Autodesk Inventor part; units mm, degrees
ref_plane "YZ Plane" through (0, 0, 0) normal (1, 0, 0) x (0, 1, 0)
ref_plane "XZ Plane" through (0, 0, 0) normal (0, 1, 0) x (-1, 0, 0)
ref_plane "XY Plane" through (0, 0, 0) normal (0, 0, 1) x (1, 0, 0)
sketch "Sketch1" plane through (0, 0, 0) normal (0, 1, 0) x (-1, 0, 0)
  line L0 (-21, 21) -> (21, 21)
  line L1 (21, 21) -> (21, -21)
  line L2 (21, -21) -> (-21, -21)
  line L3 (-21, -21) -> (-21, 21)
  line L4 (-21, 21) -> (21, -21) construction
  line L5 (21, 21) -> (-21, -21) construction
  point P0 (0, 0)
  dimension "d0" = 42
  dimension "d1" = 42
extrude "Extrusion1" add sketch "Sketch1" along normal blind 3
sketch "Sketch2" plane through (0, 3, 0) normal (0, 1, 0) x (1, 0, 0)
  circle A0 centre (0, 0) radius 3
  circle A1 centre (-15.5, -15.5) radius 1.8
  circle A2 centre (-15.5, 15.5) radius 1.8
  circle A3 centre (15.5, 15.5) radius 1.8
  circle A4 centre (15.5, -15.5) radius 1.8
  dimension "d4" = 6
  dimension "d5" = 3.6
  dimension "d6" = 31
  dimension "d7" = 15.5
  dimension "d8" = 15.5
  dimension "d9" = 31
extrude "Extrusion2" cut sketch "Sketch2" against normal blind 10
sketch "Sketch3" plane through (0, 3, 0) normal (0, 1, 0) x (1, 0, 0)
  circle A0 centre (-15.5, -15.5) radius 1.8
  circle A1 centre (-15.5, -15.5) radius 3.5
  circle A2 centre (0, 0) radius 19.3
  line L0 (-13.0251, -17.9749) -> (-10.946, -15.8958)
  line L1 (-17.9749, -13.0251) -> (-15.8958, -10.946)
  circle A3 centre (15.5, -15.5) radius 1.8
  circle A4 centre (15.5, -15.5) radius 3.5
  circle A5 centre (15.5, 15.5) radius 1.8
  circle A6 centre (15.5, 15.5) radius 3.5
  circle A7 centre (-15.5, 15.5) radius 1.8
  circle A8 centre (-15.5, 15.5) radius 3.5
  line L2 (13.0251, -17.9749) -> (10.946, -15.8958)
  line L3 (17.9749, -13.0251) -> (15.8958, -10.946)
  line L4 (13.0251, 17.9749) -> (10.946, 15.8958)
  line L5 (17.9749, 13.0251) -> (15.8958, 10.946)
  line L6 (-15.8958, 10.946) -> (-17.9749, 13.0251)
  line L7 (-10.946, 15.8958) -> (-13.0251, 17.9749)
  circle A9 centre (15.5, 15.5) radius 1.8
  circle A10 centre (-15.5, 15.5) radius 1.8
  circle A11 centre (15.5, -15.5) radius 1.8
  circle A12 centre (-15.5, -15.5) radius 1.8
  circle A13 centre (0, 0) radius 3
  line L8 (-21, 21) -> (-21, -21)
  line L9 (-21, -21) -> (21, -21)
  line L10 (21, -21) -> (21, 21)
  line L11 (21, 21) -> (-21, 21)
  dimension "d13" = 38.6
  dimension "d12" = 7
extrude "Extrusion3" cut sketch "Sketch3" against normal blind 10 contours L11 L10 L9 L8
sketch "Sketch4" plane through (0, 3, 0) normal (0, 1, 0) x (1, 0, 0)
  circle A0 centre (0, 0) radius 3
  circle A1 centre (0, 0) radius 16.125
  circle A2 centre (0, 0) radius 13.125
  dimension "d16" = 32.25
  dimension "d17" = 3
extrude "Extrusion4" add sketch "Sketch4" along normal blind 3 contours A1
fillet "Fillet1" radius 4 8 edges at (-15.8958, 1.5, -10.946) (-15.8958, 1.5, 10.946) (-10.946, 1.5, 15.8958) (10.946, 1.5, 15.8958) (15.8958, 1.5, 10.946) (15.8958, 1.5, -10.946) (10.946, 1.5, -15.8958) (-10.946, 1.5, -15.8958)
properties part number "Lid"
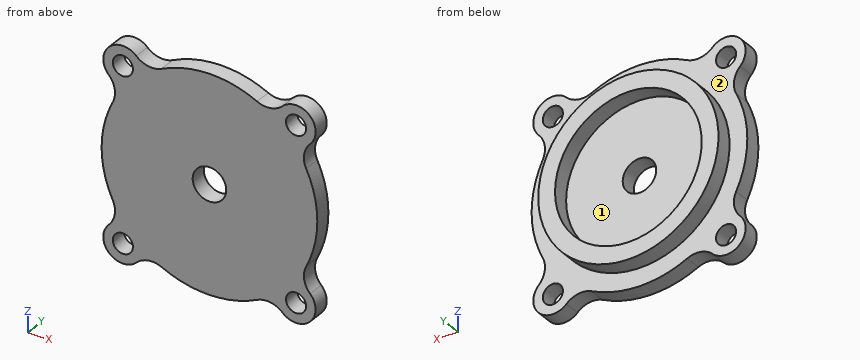
Work out the finished part from the listing and answer in its coordinate system (mm). Face numbers are marked on the shaded views. Coordinates: 2 decimals unless noted, no trailing zeros. Loops run counter-clockwise (first coordinate to the right, second up) from the corner with the lowest first, then second, coordinate; pieces in that order, holes last.
1) Consider probe 1 along X at (y, z) = (1.9, -15.5); probe 2 along X at (y, z) = (5.15, 0) (3 decimals). Determine where each line is inside the solid, lowest interval first.
Results:
probe 1: x = -19 to -17.3, -13.7 to 13.7, 17.3 to 19
probe 2: x = -16.125 to -13.125, 13.125 to 16.125
2) For a pull along Z with two mould halves and no side action, classify the marked faces 1 and 2 as +Z half, -Z half, draft (parallel to the pull), parting line (faces both ways), or undercut.
Results:
face 1: undercut
face 2: draft
3) Section D-D (x = 15.5) is taken. Give the vertices of the cut face in (y, z).
Results:
outline: (0, -19) - (3, -19) - (3, -17.3) - (0, -17.3) - close; (0, -13.7) - (3, -13.7) - (3, -4.45) - (6, -4.45) - (6, 4.45) - (3, 4.45) - (3, 13.7) - (0, 13.7) - close; (0, 17.3) - (3, 17.3) - (3, 19) - (0, 19) - close
4) Flat-ended cylindrical pins translate along their axes: pin 1 (8 mm diameter, centred on x = 5, z = 3.5, fed in from +Y); pin 2 (1.5 mm diameter, centred on y = 3, z = 13.5, fed in from +X); pin 3 (3 mm diameter, centred on x = 15.5, z = -15.5, fed in from +Y); pin 4 (1.5 mm diameter, centred on y = 4.5, z = -12, fed in from -X). Find the tip coordinate at first contact, or state that the pin passes through.
Results:
pin 1: stops at y = 3
pin 2: stops at x = 18.77
pin 3: passes through
pin 4: stops at x = -11.55
5) Section A-A (x = 0) is taken. Give the vertices of the cut face in (y, z) (3 decimals).
Results:
outline: (0, -19.3) - (3, -19.3) - (3, -16.125) - (6, -16.125) - (6, -13.125) - (3, -13.125) - (3, -3) - (0, -3) - close; (0, 3) - (3, 3) - (3, 13.125) - (6, 13.125) - (6, 16.125) - (3, 16.125) - (3, 19.3) - (0, 19.3) - close
6) Section C-C (z = -15) is taken. Give the vertices of the cut face in (x, y), plus the area to 3 significant figures.
Results:
outline: (-18.96, 0) - (-17.23, 0) - (-17.23, 3) - (-18.96, 3) - close; (-13.77, 0) - (13.77, 0) - (13.77, 3) - (5.92, 3) - (5.92, 6) - (-5.92, 6) - (-5.92, 3) - (-13.77, 3) - close; (17.23, 0) - (18.96, 0) - (18.96, 3) - (17.23, 3) - close
area: 129 mm2
7) Section B-B (z = 0) is taken. Give the vertices of the cut face in (x, y) (3 decimals).
Results:
outline: (-19.3, 0) - (-3, 0) - (-3, 3) - (-13.125, 3) - (-13.125, 6) - (-16.125, 6) - (-16.125, 3) - (-19.3, 3) - close; (3, 0) - (19.3, 0) - (19.3, 3) - (16.125, 3) - (16.125, 6) - (13.125, 6) - (13.125, 3) - (3, 3) - close
